from build123d import *

# Parameters (mm, degrees)
BASE_FLANGE1_DEPTH = 170
FILLET1_R          = 5
SKETCH6_R          = 2
CUT_EXTRUDE1_DEPTH = 178.200451467
SKETCH7_R          = 2.5
CUT_EXTRUDE2_DEPTH = 178.200451467
CUT_EXTRUDE3_DEPTH = 178.200451467
FILLET2_R          = 5
CUT_EXTRUDE4_DEPTH = 175.263907966
FILLET3_R          = 3
FILLET4_R          = 7


# Sheet-metal steps are written as plain solids
with BuildPart() as part:
    # Sketch1 → Base-Flange1 (new body)
    with BuildSketch(Plane.XY):
        with BuildLine():
            Line((0, 0), (-25.825, 0))
            ThreePointArc((-25.825, 0), (-28.777170811, 1.222829189), (-30, 4.175))
            Line((-30, 4.175), (-30, 40))
            Line((-30, 40), (-26.825, 40))
            Line((-26.825, 40), (-26.825, 4.175))
            ThreePointArc((-26.825, 4.175), (-26.532106781, 3.467893219), (-25.825, 3.175))
            Line((-25.825, 3.175), (0, 3.175))
            Line((0, 3.175), (0, 0))
        make_face()
    extrude(amount=BASE_FLANGE1_DEPTH)

    # Fillet1
    fillet1_edges = [part.edges().sort_by_distance(p)[0] for p in [
        (0, 1.5875, 170),
        (0, 1.5875, 0),
        (-28.4125, 40, 170),
        (-28.4125, 40, 0),
    ]]
    fillet(fillet1_edges, radius=FILLET1_R)

    # Sketch6 → Cut-Extrude1 (cut, through all)
    with BuildSketch(Plane.ZY.offset(30)):
        with Locations((5, 9.175)):
            Circle(SKETCH6_R)
        with BuildLine():
            ThreePointArc((159.9, 9.175), (159.835005505, 13.661766133), (159.640076561, 18.14476706))
            ThreePointArc((159.640076561, 18.14476706), (156.999504521, 20.49580498), (154.648466601, 17.85523294))
            ThreePointArc((154.648466601, 17.85523294), (154.837103455, 13.516938304), (154.9, 9.175))
            ThreePointArc((154.9, 9.175), (157.4, 6.675), (159.9, 9.175))
        make_face()
    extrude(amount=-CUT_EXTRUDE1_DEPTH, mode=Mode.SUBTRACT)

    # Sketch7 → Cut-Extrude2 (cut, through all)
    with BuildSketch(Plane.XZ):
        with Locations(Location((-15.4125, 160, 0), (0, 0, 270))):
            Circle(SKETCH7_R)
        with Locations(Location((-15.4125, 85, 0), (0, 0, 270))):
            Circle(SKETCH7_R)
        with Locations(Location((-15.4125, 10, 0), (0, 0, 270))):
            Circle(SKETCH7_R)
    extrude(amount=-CUT_EXTRUDE2_DEPTH, mode=Mode.SUBTRACT)

    # Sketch8 → Cut-Extrude3 (cut, through all)
    with BuildSketch(Plane.ZY.offset(30)):
        with BuildLine():
            Line((0, 12.85080004), (170, 24.175))
            Line((170, 24.175), (170, 35))
            ThreePointArc((170, 35), (168.535533906, 38.535533906), (165, 40))
            Line((165, 40), (5, 40))
            ThreePointArc((5, 40), (1.464466094, 38.535533906), (0, 35))
            Line((0, 35), (0, 12.85080004))
        make_face()
    extrude(amount=-CUT_EXTRUDE3_DEPTH, mode=Mode.SUBTRACT)

    # Fillet2
    fillet2_edges = [part.edges().sort_by_distance(p)[0] for p in [
        (-28.4125, 24.175, 170),
        (-28.4125, 12.85080004, 0),
    ]]
    fillet(fillet2_edges, radius=FILLET2_R)

    # Sketch9 → Cut-Extrude4 (cut, through all)
    with BuildSketch(Plane.ZY.offset(30)):
        Polygon((10, 13.51692945), (10, 4.175), (145, 4.175), (145, 22.509676476), align=None)
    extrude(amount=-CUT_EXTRUDE4_DEPTH, mode=Mode.SUBTRACT)

    # Fillet3
    fillet3_edges = [part.edges().sort_by_distance(p)[0] for p in [
        (-28.4125, 4.175, 10),
        (-28.4125, 13.51692945, 10),
    ]]
    fillet(fillet3_edges, radius=FILLET3_R)

    # Fillet4
    fillet4_edges = [part.edges().sort_by_distance(p)[0] for p in [
        (-28.4125, 22.509676476, 145),
        (-28.4125, 4.175, 145),
    ]]
    fillet(fillet4_edges, radius=FILLET4_R)


solid = part.part
Work out the finished part from the listing and answer in its coordinate system (mm). A direction names the side the tool comes from. Give positions to 0.01 mm unless a question says otherwise; leave off trailing zeros. Write each loop counter-clockwise with the first axis right and the second up, starting at its lowest first coordinate (ties: lowest second). Pieces come first, ordered by that corner, then holes. Notation, with made-up numbers: (-31.5, -23) - (-14.5, -23) arc R25 cw to (-14.5, 9) - close; hole circle Ø2 at (78, 44.25). An arc over 180 degrees is marked (long way). One line per item, written item: value. Start each with the question number.
1. Find section B-B (z = 114.5). Write down the section's boundary in (x, y) (3 decimals).
2. Consider probe 1 along Y at (x, z) = (-6.5, 68) (3 decimals); probe 2 along X at (y, z) = (12, 9) (3 decimals); probe 3 along Y at (x, z) = (-28, 5) (3 decimals). Determine where each line is inside the solid, lowest interval first.
3. For faces 1 (the flat face through (-28, 9, 10)), 2 (the flat face through (-26.825, 7, 5)), 3 (the cylindrical face through (-28.435, 13.599, 159.837)), 4 (the flat face through (-12.7, 0, 83.8)), determine the directions among +Z, -Z, +X, -X, +Y, -Y from which every point of the face is accessible in a straight line to the end or side of a thin tool.
4. Given pin 1 (10 mm diameter, centred on x = -20.5, y = 18, fed in from -Z); pin 2 (6 mm diameter, centred on y = 11.5, z = 155, fed in from +X) (3 decimals); pin 3 (5 mm diameter, centred on y = 9.175, z = 5, fed in from -X); pin 4 (1 mm diameter, centred on x = -28, y = 13, fed in from -Z), each flat-ended and moving along its own axis, determine where each tip first touches the part or whether it passes through.
5. Find section C-C (x = -8.5). Write down the section's boundary in (y, z) (3 decimals).
6. For a pull along Z with two mould halves and no side action, classify faces 5 (the flat face through (-28, 4.175, 75)), 6 (the flat face through (-10, 3.175, 84)), 7 (the flat face through (-28.435, 23.376, 158.009)) as +Z half, -Z half, draft (parallel to the pull), parting line (faces both ways), or undercut.
Geometry results:
1. outline: (-30, 4.175) arc R4.175 ccw to (-25.825, 0) - (0, 0) - (0, 3.175) - (-25.825, 3.175) arc R1 cw to (-26.825, 4.175) - close
2. probe 1: 0 to 3.175
2. probe 2: -30 to -26.825
2. probe 3: 0.611 to 7.175, 11.175 to 13.184
3. face 1: +X, -X, +Y
3. face 2: +Z, -Z, +X, +Y
3. face 3: +X, -X
3. face 4: +Z, -Z, +X, -X, -Y
4. pin 1: through
4. pin 2: x = -26.825
4. pin 3: x = -30
4. pin 4: z = 2.49
5. outline: (0, 0) - (3.175, 0) - (3.175, 170) - (0, 170) - close
6. face 5: undercut
6. face 6: draft
6. face 7: -Z half
